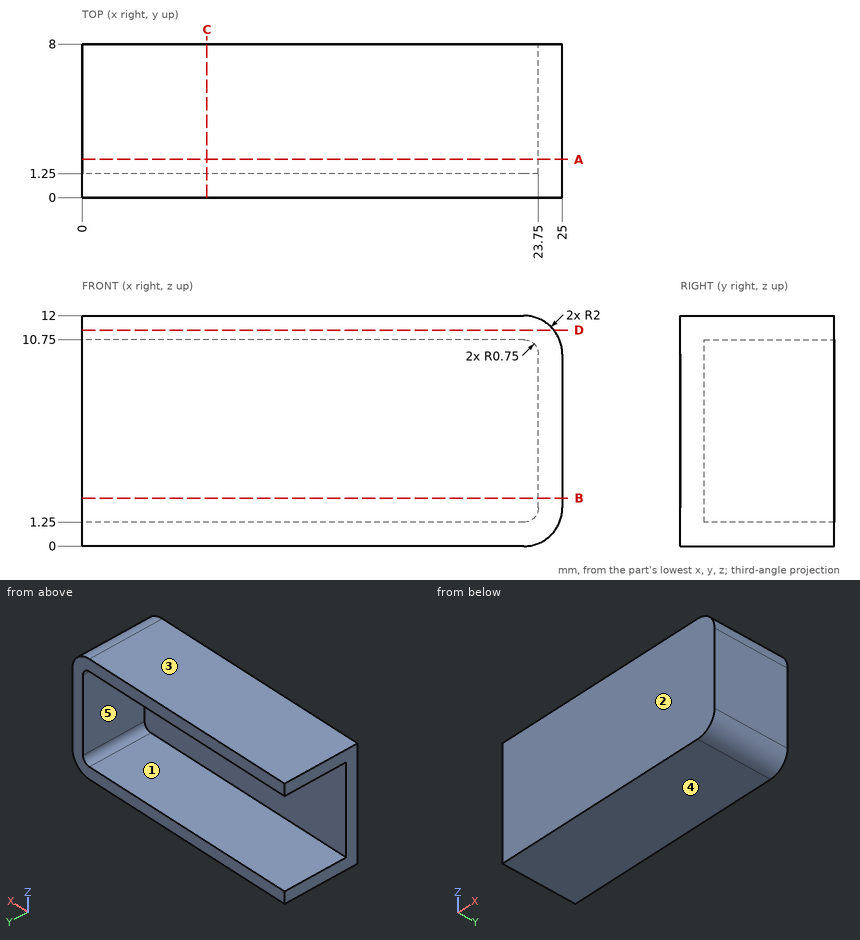
Here's the drawing with two shaded views (mm, measured from the low corner). I have some questions. A direction names the side the tool comes from. Give positions to 0.01 mm unless a question says otherwise; leave off trailing zeros. Loops run counter-clockwise (first coordinate to the right, second up) from the corner with the lowest first, then second, coordinate; pieces in that order, holes last. Notation, with made-up numbers: (74.5, -34) -> (126.5, -34) arc R13 cw to (126.5, -11) -> close; hole circle Ø4 at (30, -29.75). An arc over 180 degrees is marked (long way). Answer as a JSON object with one key per item and string values. Group by question number.
Item 1: I need wall thicknesses on L1, parallel to Z at x = 21.75, y = 1.75; L2, parallel to X at y = 4.75, z = 5.5; L3, parallel to Y at x = 7, z = 9.5. Which ranges of each line are inside material? Lowest first, please.
Item 2: Imagine slicing it at D-D on z = 11.25. Write out the boundary of the cut face in (x, y), then the cut area to 3 significant figures.
Item 3: On a 3-axis mill with a long thin cutter (end or side, diameter ignored), from which of +Z, -Z, +X, -X, +Y, -Y can I reach the whole of each face in a straight line? I mean the marked faces 4 and 5. Say none if no direction works.
Item 4: Will this pin go through, and if not, where does the flat tip stop? pin 1 (1.5 mm diameter, centred on y = 5.5, z = 5, fed in from -X).
Item 5: Imagine slicing it at A-A on y = 2. Write out the boundary of the cut face in (x, z), then the cut area to 3 significant figures.
Item 6: Thinking about a two-plate mould opening in Z: for the marked faces 1, 2 and 3, which applies, pulls with the +Z half, pulls with the -Z half, needs draft (parallel to the pull), parting line crosses it, or undercut?
Item 7: Imagine slicing it at B-B on z = 2.5. Write out the boundary of the cut face in (x, y), then the cut area to 3 significant figures.
Item 8: Imagine slicing it at C-C on x = 6.5. Write out the boundary of the cut face in (y, z).
Answer list:
{
 "1": {"L1": "z = 0 to 1.25, 10.75 to 12", "L2": "x = 23.75 to 25", "L3": "y = 0 to 1.25"},
 "2": {"outline": "(0, 0) -> (24.56, 0) -> (24.56, 8) -> (0, 8) -> close", "area": "196 mm2"},
 "3": {"face 4": "-Z, +X, -X, +Y, -Y", "face 5": "-X, +Y"},
 "4": {"pin 1": "stops at x = 23.75"},
 "5": {"outline": "(0, 0) -> (23, 0) arc R2 ccw to (25, 2) -> (25, 10) arc R2 ccw to (23, 12) -> (0, 12) -> (0, 10.75) -> (23, 10.75) arc R0.75 cw to (23.75, 10) -> (23.75, 2) arc R0.75 cw to (23, 1.25) -> (0, 1.25) -> close", "area": "72.9 mm2"},
 "6": {"face 1": "undercut", "face 2": "needs draft", "face 3": "pulls with the +Z half"},
 "7": {"outline": "(0, 0) -> (25, 0) -> (25, 8) -> (23.75, 8) -> (23.75, 1.25) -> (0, 1.25) -> close", "area": "39.7 mm2"},
 "8": {"outline": "(0, 0) -> (8, 0) -> (8, 1.25) -> (1.25, 1.25) -> (1.25, 10.75) -> (8, 10.75) -> (8, 12) -> (0, 12) -> close"}
}
